from build123d import *

# Parameters (mm, degrees)
F0_W     = 39.875954
F0_H     = 91.495306
F1_DEPTH = 16.51
F2_R     = 9.901049
F3_DEPTH = 39.878
F4_W     = 19.099163
F4_H     = 47.554333
F5_DEPTH = 25.4


with BuildPart() as f1:
    # F0 (on Front) → F1 (new body)
    with BuildSketch(Plane.XZ):
        Rectangle(F0_W, F0_H)
    extrude(amount=-F1_DEPTH)

    # F2 (on face) → F3 (cut)
    with BuildSketch(Plane.XZ):
        Circle(F2_R)
    extrude(amount=-F3_DEPTH, mode=Mode.SUBTRACT)

    # F4 (on Front) → F5 (cut)
    with BuildSketch(Plane.XZ):
        with Locations((0.064525, 23.777166)):
            Rectangle(F4_W, F4_H)
    extrude(amount=-F5_DEPTH, mode=Mode.SUBTRACT)


solid = f1.part
The listing builds one solid part. Answer for the finished solid, in the listing's coordinates (mm). A direction names the side the tool comes from. Round coordinates to 2 decimals unless told otherwise and drop trailing zeros. Order: outer loops, then holes, each group sorted by start corner. A loop starts at its lowest first (then second) coordinate and runs counter-clockwise, first axis right, second up. Notation, with made-up numbers: (56.5, -16.5) -> (75.5, -16.5) arc R26 ccw to (75.5, 7.5) -> close; hole circle Ø10 at (32.5, 54.5). An arc over 180 degrees is marked (long way). One line per item, written item: value.
Item 1: Find section A-A, the plane z = 16. Give the vertices of the cut face in (x, y), then the cut area to 3 significant figures.
Taken from the geometry:
outline: (-19.94, 0) -> (-9.49, 0) -> (-9.49, 16.51) -> (-19.94, 16.51) -> close; (9.61, 0) -> (19.94, 0) -> (19.94, 16.51) -> (9.61, 16.51) -> close
area: 343 mm2
Item 2: For faces 4 (the flat face through (9.614, 8, 24)), 5 (the flat face through (-15, 8, 45.748)), determine the directions among +Z, -Z, +X, -X, +Y, -Y from which every point of the face is accessible in a straight line to the end or side of a thin tool.
Taken from the geometry:
face 4: +Z, +Y, -Y
face 5: +Z, +X, -X, +Y, -Y
Item 3: Straight lines are drawn through the part: L1, parallel to X at y = 5.25, z = 0; L2, parallel to X at y = 2, z = 18; L3, parallel to Z at x = 0, y = 9.75. For each, find the intervals that lie inside material, in ascending order.
Taken from the geometry:
L1: x = -19.94 to -9.9, 9.9 to 19.94
L2: x = -19.94 to -9.49, 9.61 to 19.94
L3: z = -45.75 to -9.9
Item 4: Find section D-D, the plane z = 0. Give the vertices of the cut face in (x, y), then the cut area to 3 significant figures.
Taken from the geometry:
outline: (-19.94, 0) -> (-9.9, 0) -> (-9.9, 16.51) -> (-19.94, 16.51) -> close; (9.9, 0) -> (19.94, 0) -> (19.94, 16.51) -> (9.9, 16.51) -> close
area: 331 mm2
Item 5: Given P1, Ø1, axis at x = -2.5, y = 12, coming from the +Z side, flat-ended and moving along its own axis, determine where the tip first touches the part or whether it passes through.
Taken from the geometry:
P1: stops at z = -9.44
Item 6: Find section B-B, the plane y = 7.5. Give the vertices of the cut face in (x, z).
Taken from the geometry:
outline: (-19.94, -45.75) -> (19.94, -45.75) -> (19.94, 45.75) -> (9.61, 45.75) -> (9.61, 2.37) arc R9.9 cw (long way) to (-9.49, 2.84) -> (-9.49, 45.75) -> (-19.94, 45.75) -> close
Item 7: Find section C-C, the plane x = 0. Give the vertices of the cut face in (y, z).
Taken from the geometry:
outline: (0, -45.75) -> (16.51, -45.75) -> (16.51, -9.9) -> (0, -9.9) -> close
Item 8: For a pull along X with two mould halves and no side action, classify faces 1 (the flat face through (19.938, 8, -1)), 2 (the cylindrical face through (-0.5, 8.14, -9.89)), 3 (the flat face through (-5, 0, -10)) as released by +X, released by -X, zero draft, split by the parting line, or undercut.
Taken from the geometry:
face 1: released by +X
face 2: undercut
face 3: zero draft
